Geometry check sheet. Reference: the model listing, model coordinates, mm. Face numbers are marked on the shaded views. A direction names the side the tool comes from. Give positions to 0.01 mm unless a question says otherwise; leave off trailing zeros. Order: outer loops, then holes, each group sorted by start corner. A loop starts at its lowest first (then second) coordinate and runs counter-clockwise, first axis right, second up. Notation, with made-up numbers: M 74.25,43.5 L 99.25,43.5 A14 cw 99.25,62.5 Z; hole C -35.75,-17.5 d11. An arc over 180 degrees is marked long. Answer as CSV lines item,"result". Start each with the question number.
```python
from build123d import *

# Parameters (mm, degrees)
SALIENTE_EXTRUIR1_DEPTH  = 3
SALIENTE_EXTRUIR3_DEPTH  = 6
SALIENTE_EXTRUIR4_DEPTH  = 2
SALIENTE_EXTRUIR5_DEPTH  = 2
REDONDEO1_R              = 3
CROQUIS5_R               = 1
CORTAR_EXTRUIR1_DEPTH    = 5
CORTAR_EXTRUIR2_START    = -5
CROQUIS6_R               = 1
CORTAR_EXTRUIR2_DEPTH    = 5
SALIENTE_EXTRUIR6_START  = -5
SALIENTE_EXTRUIR6_DEPTH  = 5
CROQUIS9_W               = 22.939215458
CROQUIS9_H               = 15.240437668
CORTAR_EXTRUIR3_DEPTH    = 8
REDONDEO2_R              = 3
SALIENTE_EXTRUIR13_DEPTH = 2
SALIENTE_EXTRUIR15_DEPTH = 2


with BuildPart() as part:
    # Croquis1 → Saliente-Extruir1 (new body)
    with BuildSketch(Plane(origin=(0, 0, 0), x_dir=(1, 0, 0), z_dir=(0, 1, 0))):
        with BuildLine():
            Line((-15.85, -12.95), (15.85, -12.95))
            ThreePointArc((15.85, -12.95), (18.678427125, -11.778427125), (19.85, -8.95))
            Line((19.85, -8.95), (19.85, 8.95))
            ThreePointArc((19.85, 8.95), (18.678427125, 11.778427125), (15.85, 12.95))
            Line((15.85, 12.95), (-15.85, 12.95))
            ThreePointArc((-15.85, 12.95), (-18.678427125, 11.778427125), (-19.85, 8.95))
            Line((-19.85, 8.95), (-19.85, -8.95))
            ThreePointArc((-19.85, -8.95), (-18.678427125, -11.778427125), (-15.85, -12.95))
        make_face()
    extrude(amount=SALIENTE_EXTRUIR1_DEPTH)

    # Croquis2 → Saliente-Extruir3 (add)
    with BuildSketch(Plane(origin=(0, 3, 0), x_dir=(1, 0, 0), z_dir=(0, 1, 0))):
        with BuildLine():
            Line((-15.85, -10.95), (15.85, -10.95))
            ThreePointArc((15.85, -10.95), (17.264213562, -10.364213562), (17.85, -8.95))
            Line((17.85, -8.95), (17.85, 8.95))
            ThreePointArc((17.85, 8.95), (17.264213562, 10.364213562), (15.85, 10.95))
            Line((15.85, 10.95), (-15.85, 10.95))
            ThreePointArc((-15.85, 10.95), (-17.264213562, 10.364213562), (-17.85, 8.95))
            Line((-17.85, 8.95), (-17.85, -8.95))
            ThreePointArc((-17.85, -8.95), (-17.264213562, -10.364213562), (-15.85, -10.95))
        make_face()
    extrude(amount=SALIENTE_EXTRUIR3_DEPTH)

    # Croquis3 → Saliente-Extruir4 (add)
    with BuildSketch(Plane(origin=(0, 9, 0), x_dir=(1, 0, 0), z_dir=(0, 1, 0))):
        with BuildLine():
            Line((-15.85, -9.45), (15.85, -9.45))
            ThreePointArc((15.85, -9.45), (16.203553391, -9.303553391), (16.35, -8.95))
            Line((16.35, -8.95), (16.35, 8.95))
            ThreePointArc((16.35, 8.95), (16.203553391, 9.303553391), (15.85, 9.45))
            Line((15.85, 9.45), (-15.85, 9.45))
            ThreePointArc((-15.85, 9.45), (-16.203553391, 9.303553391), (-16.35, 8.95))
            Line((-16.35, 8.95), (-16.35, -8.95))
            ThreePointArc((-16.35, -8.95), (-16.203553391, -9.303553391), (-15.85, -9.45))
        make_face()
    extrude(amount=SALIENTE_EXTRUIR4_DEPTH)

    # Croquis4 → Saliente-Extruir5 (add)
    with BuildSketch(Plane(origin=(0, 11, 0), x_dir=(1, 0, 0), z_dir=(0, 1, 0))):
        with BuildLine():
            Line((-15.85, -10.95), (15.85, -10.95))
            ThreePointArc((15.85, -10.95), (17.264213562, -10.364213562), (17.85, -8.95))
            Line((17.85, -8.95), (17.85, 8.95))
            ThreePointArc((17.85, 8.95), (17.264213562, 10.364213562), (15.85, 10.95))
            Line((15.85, 10.95), (-15.85, 10.95))
            ThreePointArc((-15.85, 10.95), (-17.264213562, 10.364213562), (-17.85, 8.95))
            Line((-17.85, 8.95), (-17.85, -8.95))
            ThreePointArc((-17.85, -8.95), (-17.264213562, -10.364213562), (-15.85, -10.95))
        make_face()
    extrude(amount=SALIENTE_EXTRUIR5_DEPTH)

    # Redondeo1
    redondeo1_edges = [part.edges().sort_by_distance(p)[0] for p in [
        (0, 0, -12.95),
        (-18.678427125, 0, -11.778427125),
        (-19.85, 0, 0),
        (-18.678427125, 0, 11.778427125),
        (0, 0, 12.95),
        (18.678427125, 0, 11.778427125),
        (19.85, 0, 0),
        (18.678427125, 0, -11.778427125),
    ]]
    fillet(redondeo1_edges, radius=REDONDEO1_R - 0.0001)  # a hair under: the kernel refuses the full size

    # Croquis5 → Cortar-Extruir1 (cut)
    with BuildSketch(Plane.ZY.offset(17.85)):
        with Locations((0, 6)):
            Circle(CROQUIS5_R)
    extrude(amount=-CORTAR_EXTRUIR1_DEPTH, mode=Mode.SUBTRACT)

    # Croquis6 → Cortar-Extruir2 (cut)
    with BuildSketch(Plane(origin=(17.85, 0, 0), x_dir=(0, 0, -1), z_dir=(1, 0, 0)).offset(CORTAR_EXTRUIR2_START)):
        with Locations(Location((0, 6, 0), (0, 0, 180))):
            Circle(CROQUIS6_R)
    extrude(amount=CORTAR_EXTRUIR2_DEPTH, mode=Mode.SUBTRACT)

    # Croquis8 → Saliente-Extruir6 (add)
    with BuildSketch(Plane(origin=(0, 13, 0), x_dir=(1, 0, 0), z_dir=(0, 1, 0)).offset(SALIENTE_EXTRUIR6_START)):
        with BuildLine():
            ThreePointArc((16.35, 8.95), (16.287739315, 9.387739315), (15.85, 9.45))
            ThreePointArc((15.85, 9.45), (16.203553391, 9.303553391), (16.35, 8.95))
        make_face()
        with BuildLine():
            ThreePointArc((15.85, -9.45), (16.203553391, -9.303553391), (16.35, -8.95))
            ThreePointArc((16.35, -8.95), (16.287739315, -9.387739315), (15.85, -9.45))
        make_face()
        with BuildLine():
            ThreePointArc((-16.35, -8.95), (-16.203553391, -9.303553391), (-15.85, -9.45))
            ThreePointArc((-15.85, -9.45), (-16.287739315, -9.387739315), (-16.35, -8.95))
        make_face()
        with BuildLine():
            ThreePointArc((-16.35, 8.95), (-16.287739315, 9.387739315), (-15.85, 9.45))
            ThreePointArc((-15.85, 9.45), (-16.203553391, 9.303553391), (-16.35, 8.95))
        make_face()
    extrude(amount=SALIENTE_EXTRUIR6_DEPTH)

    # Croquis9 → Cortar-Extruir3 (cut)
    with BuildSketch(Plane(origin=(0, 13, 0), x_dir=(1, 0, 0), z_dir=(0, 1, 0))):
        with Locations((0.209490552, 0.130931595)):
            Rectangle(CROQUIS9_W, CROQUIS9_H)
    extrude(amount=-CORTAR_EXTRUIR3_DEPTH, mode=Mode.SUBTRACT)

    # Redondeo2
    redondeo2_edges = [part.edges().sort_by_distance(p)[0] for p in [
        (11.679098281, 9, 7.489287239),
        (-11.260117177, 9, 7.489287239),
        (-11.260117177, 9, -7.751150429),
        (11.679098281, 9, -7.751150429),
    ]]
    fillet(redondeo2_edges, radius=REDONDEO2_R)

    # Croquis11 → Saliente-Extruir13 (add)
    with BuildSketch(Plane(origin=(0, 9, 0), x_dir=(1, 0, 0), z_dir=(0, 1, 0))):
        with BuildLine():
            Line((-16.35, -8.95), (-16.35, -8.722324592))
            ThreePointArc((-16.35, -8.722324592), (-16.402564717, -9.58947242), (-15.545094105, -9.45))
            Line((-15.545094105, -9.45), (-15.85, -9.45))
            ThreePointArc((-15.85, -9.45), (-16.287739315, -9.387739315), (-16.35, -8.95))
        make_face()
        with BuildLine():
            ThreePointArc((16.35, 8.722324592), (16.402564717, 9.58947242), (15.545094105, 9.45))
            Line((15.545094105, 9.45), (15.85, 9.45))
            ThreePointArc((15.85, 9.45), (16.287739315, 9.387739315), (16.35, 8.95))
            Line((16.35, 8.95), (16.35, 8.722324592))
        make_face()
        with BuildLine():
            Line((15.85, -9.45), (15.545094105, -9.45))
            ThreePointArc((15.545094105, -9.45), (16.402564717, -9.58947242), (16.35, -8.722324592))
            Line((16.35, -8.722324592), (16.35, -8.95))
            ThreePointArc((16.35, -8.95), (16.287739315, -9.387739315), (15.85, -9.45))
        make_face()
    extrude(amount=SALIENTE_EXTRUIR13_DEPTH)

    # Croquis13 → Saliente-Extruir15 (add)
    with BuildSketch(Plane(origin=(0, 9, 0), x_dir=(1, 0, 0), z_dir=(0, 1, 0))):
        with BuildLine():
            Line((-16.35, 8.95), (-16.35, 8.457615485))
            ThreePointArc((-16.35, 8.457615485), (-16.500312948, 9.537460741), (-15.413569935, 9.45))
            Line((-15.413569935, 9.45), (-15.85, 9.45))
            ThreePointArc((-15.85, 9.45), (-16.287739315, 9.387739315), (-16.35, 8.95))
        make_face()
    extrude(amount=SALIENTE_EXTRUIR15_DEPTH)


solid = part.part
```
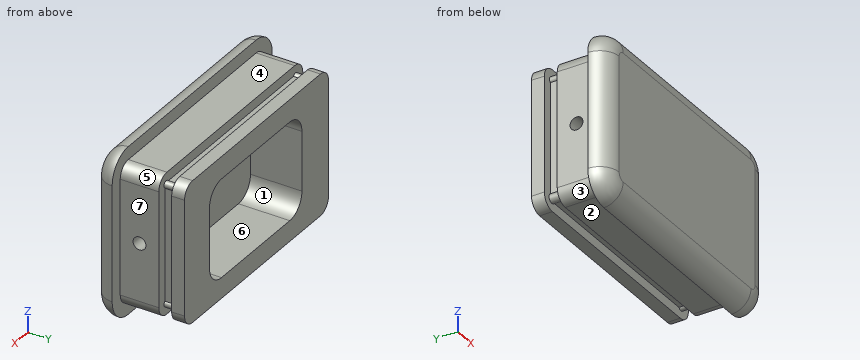
Item 1: Depth check by flat-ended pin: pin 1 Ø6.5 at (x, y) = (-4, 10.5) entering from -Z; pin 2 Ø2.5 at (y, z) = (7.5, 1) entering from -X; pin 3 Ø0.6 at (x, y) = (3, 10) entering from +Z. Enter the tip coordinate at first touch or a pass-through.
Item 2: Section check B-B on y = 6. Record the boundary of the cut face in (x, z), then the cut area to 3 significant figures.
Item 3: Access from +Z, -Z, +X, -X, +Y, -Y to the whole of each face (thin tool, end or side, straight path). Record for the marked faces 1, 2, 3 and 4.
Item 4: Draft check along Z on the marked faces 5, 6 and 7. Enter one of: pulls with the +Z half, pulls with the -Z half, needs draft (parallel to the pull), parting line crosses it, or undercut.
Item 5: Scan lines: line 1 along Z through (x, y) = (-1, 10.75); line 2 along Z through (x, y) = (0, 7.5); line 3 along Y through (x, z) = (-14, -10). Record each from-to range of solid material in increasing order.
Numbers:
1,pin 1,"z = -10.95"
1,pin 2,"x = -17.85"
1,pin 3,"z = 9.45"
2,outline,"M -17.85,-8.95 A2 ccw -15.85,-10.95 L 15.85,-10.95 A2 ccw 17.85,-8.95 L 17.85,-1 L 12.85,-1 L 12.85,1 L 17.85,1 L 17.85,8.95 A2 ccw 15.85,10.95 L -15.85,10.95 A2 ccw -17.85,8.95 L -17.85,1 L -12.85,1 L -12.85,-1 L -17.85,-1 Z; hole M -11.26,-4.75 A3 ccw -8.26,-7.75 L 8.68,-7.75 A3 ccw 11.68,-4.75 L 11.68,4.49 A3 ccw 8.68,7.49 L -8.26,7.49 A3 ccw -11.26,4.49 Z"
2,area,"417 mm2"
3,face 1,"+Y"
3,face 2,"-Z, +X, -X, +Y"
3,face 3,"-Z, -X, +Y"
3,face 4,"+Z, +X, -X, +Y"
4,face 5,"pulls with the +Z half"
4,face 6,"undercut"
4,face 7,"needs draft"
5,line 1,"-9.45 to -7.75, 7.49 to 9.45"
5,line 2,"-10.95 to -7.75, 7.49 to 10.95"
5,line 3,"0 to 9, 11 to 13"
